Read the model definition and answer for the solid it produces. Units are mm, in the model's axes. A direction names the side the tool comes from. Coordinates: 2 decimals unless noted, no trailing zeros. Write each loop counter-clockwise with the first axis right and the second up, starting at its lowest first coordinate (ties: lowest second). Pieces come first, ordered by that corner, then holes. Notation, with made-up numbers: M -39,50 L -16,50 A30 cw -16,84 Z; hole C 79,71 d5. An arc over 180 degrees is marked long. Write item = value, one per line.
from build123d import *

# Parameters (mm, degrees)
SKETCH1_W           = 24
SKETCH1_H           = 45
BOSS_EXTRUDE1_DEPTH = 3
SKETCH4_R           = 4
SKETCH4_W           = 3
SKETCH4_H           = 10
CUT_EXTRUDE1_DEPTH  = 4


with BuildPart() as part:
    # Sketch1 → Boss-Extrude1 (new body)
    with BuildSketch(Plane(origin=(0, 0, 0), x_dir=(1, 0, 0), z_dir=(0, 1, 0))):
        Rectangle(SKETCH1_W, SKETCH1_H)
    extrude(amount=BOSS_EXTRUDE1_DEPTH)

    # Sketch4 → Cut-Extrude1 (cut, through all)
    with BuildSketch(Plane(origin=(0, 3, 0), x_dir=(1, 0, 0), z_dir=(0, 1, 0))):
        with Locations((0, 14.5)):
            Circle(SKETCH4_R)
        with Locations((-10.5, -7.5)):
            Rectangle(SKETCH4_W, SKETCH4_H)
        with Locations((-10.5, 12.5)):
            Rectangle(SKETCH4_W, SKETCH4_H)
        with Locations((10.5, 12.5)):
            Rectangle(SKETCH4_W, SKETCH4_H)
        with Locations((10.5, -7.5)):
            Rectangle(SKETCH4_W, SKETCH4_H)
    extrude(amount=-CUT_EXTRUDE1_DEPTH, mode=Mode.SUBTRACT)


solid = part.part
Item 1: Find section C-C (x = 10.25). Determine the outline of the cut face in (y, z), and give its area (3 significant figures).
Worked answers:
outline = M 0,-22.5 L 3,-22.5 L 3,-17.5 L 0,-17.5 Z; M 0,-7.5 L 3,-7.5 L 3,2.5 L 0,2.5 Z; M 0,12.5 L 3,12.5 L 3,22.5 L 0,22.5 Z
area = 75.0 mm²
Item 2: Find section D-D (x = 0). Determine the outline of the cut face in (y, z), and give its area (3 significant figures).
Worked answers:
outline = M 0,-22.5 L 3,-22.5 L 3,-18.5 L 0,-18.5 Z; M 0,-10.5 L 3,-10.5 L 3,22.5 L 0,22.5 Z
area = 111 mm²
Item 3: Which of the six approach directions +Z, -Z, +X, -X, +Y, -Y give full straight-line access (tool end or side, diameter ignored) to faces 4 (the face through (-9, 2, 8)), 5 (the face through (9, 2, -12)), 6 (the face through (-12, 1, -2))?
Worked answers:
face_4 = -X, +Y, -Y
face_5 = +X, +Y, -Y
face_6 = +Z, -Z, -X, +Y, -Y
Item 4: Find section B-B (z = -14.5). Determine the outline of the cut face in (x, y).
Worked answers:
outline = M -9,0 L -4,0 L -4,3 L -9,3 Z; M 4,0 L 9,0 L 9,3 L 4,3 Z
Item 5: A flat-ended cylindrical pin translates along its axis: pin 1 (1.5 mm diameter, centred on y = 1, z = 7, fed in from +X). Find the tip coordinate at first contact, or state that the pin passes through.
Worked answers:
pin_1 = 9
Item 6: Find section A-A (y = 2.4). Determine the outline of the cut face in (x, z).
Worked answers:
outline = M -12,-22.5 L 12,-22.5 L 12,-17.5 L 9,-17.5 L 9,-7.5 L 12,-7.5 L 12,2.5 L 9,2.5 L 9,12.5 L 12,12.5 L 12,22.5 L -12,22.5 L -12,12.5 L -9,12.5 L -9,2.5 L -12,2.5 L -12,-7.5 L -9,-7.5 L -9,-17.5 L -12,-17.5 Z; hole C 0,-14.5 d8
Item 7: For a pull along X with two mould halves and no side action, classify faces 1 (the face through (-12, 1, -20)), 2 (the face through (-0.521, 1.521, -18.466)), 3 (the face through (9, 2, 8)) as released by +X, released by -X, zero draft, split by the parting line, or undercut.
Worked answers:
face_1 = released by -X
face_2 = undercut
face_3 = released by +X
Item 8: Consider line 1 along Z through (x, y) = (-10, 0.8); line 2 along Z through (x, y) = (0, 2.1); line 3 along X through (y, z) = (1.2, -14.5). Determine where each line is inside the solid, lowest interval first. Write a range as from..to.
Worked answers:
line_1 = -22.5..-17.5, -7.5..2.5, 12.5..22.5
line_2 = -22.5..-18.5, -10.5..22.5
line_3 = -9..-4, 4..9
